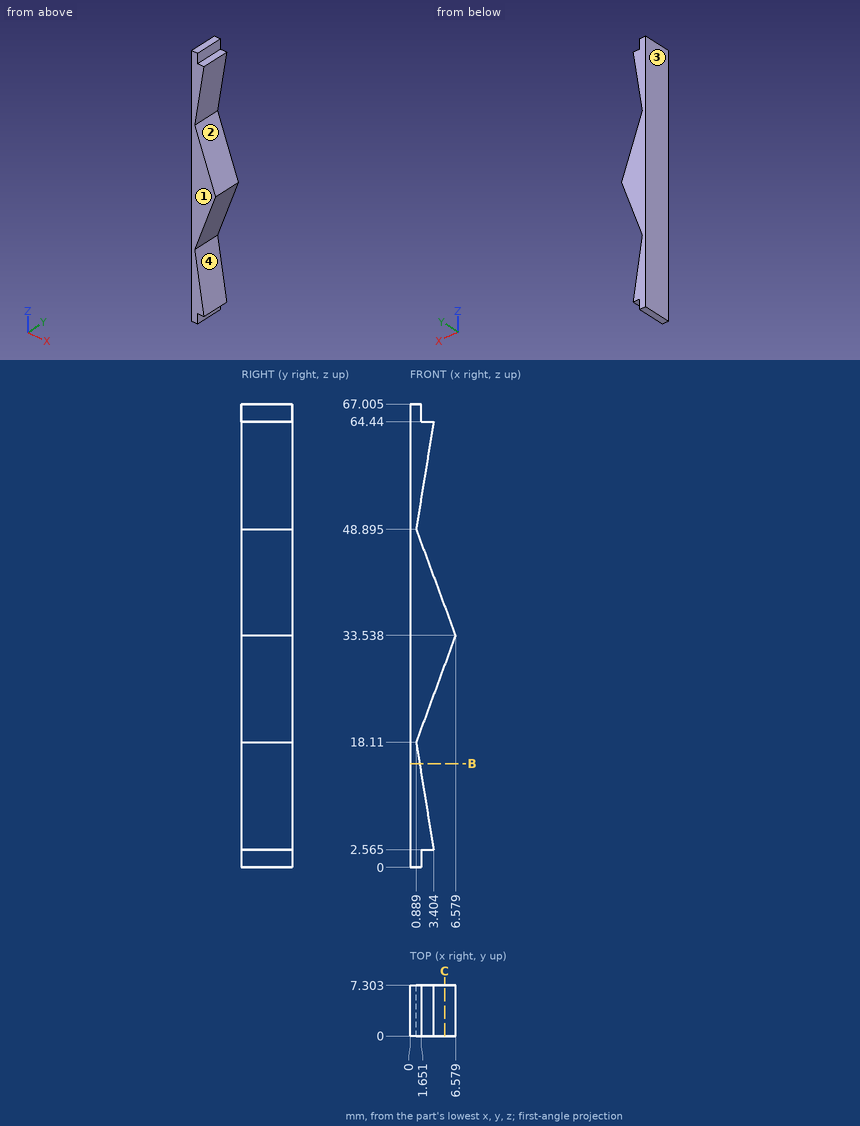
Design review of the part shown in the three views and the two pictorial views. Dimensions are in mm from the part's minimum x, y and z. A direction names the side the tool comes from. Coordinates: 2 decimals unless noted, no trailing zeros. Loops run counter-clockwise (first coordinate to the right, second up) from the corner with the lowest first, then second, coordinate; pieces in that order, holes last.
Q1. To check wall thickness, follow line 1 (X direction, y = 4.75, z = 46.5) (1 decimal); line 2 (X direction, y = 0.5, z = 39.5). State the ranges of each line that lie inside material, in increasing order.
Reported:
line 1: x = 0 to 1.8
line 2: x = 0 to 4.37
Q2. The part is to be moulded in two halves that separate along Z. For the marked faces 1 and 2, say which applies: +Z half, -Z half, draft (parallel to the pull), parting line (faces both ways), or undercut.
Reported:
face 1: draft
face 2: undercut
Q3. For pin 1 (1.5 mm diameter, centred on y = 3.5, z = 54, fed in from +X); pin 2 (0.8 mm diameter, centred on y = 4.5, z = 66, fed in from +X); pin 3 (0.5 mm diameter, centred on x = 2, y = 4, fed in from -Z) (1 decimal); pin 4 (1.9 mm diameter, centred on x = 2.5, y = 3.5, fed in from +Z) (1 decimal), all flat-tipped, find the tip position at first contact; note any pin that passes through.
Reported:
pin 1: stops at x = 1.84
pin 2: stops at x = 1.65
pin 3: stops at z = 2.6
pin 4: stops at z = 67
Q4. We need section C-C on x = 5. State the section outline as (y, z) points.
Reported:
outline: (0, 29.26) - (7.3, 29.26) - (7.3, 37.8) - (0, 37.8) - close
Q5. We need section B-B on z = 15. State the section outline as (x, y) points.
Reported:
outline: (0, 0) - (1.39, 0) - (1.39, 7.3) - (0, 7.3) - close
Q6. Tool access review of the marked faces 3 and 4: name each direction out of +Z, -Z, +X, -X, +Y, -Y from which nothing blocks a thin tool from reaching the whole face with its end or side.
Reported:
face 3: +Z, -Z, -X, +Y, -Y
face 4: +X, +Y, -Y
